Check sheet for the drawn part. Datum: minimum x, y, z corner. Units: mm. Round coordinates to 2 decimals unless told otherwise and drop trailing zeros. Order: outer loops, then holes, each group sorted by start corner. A loop starts at its lowest first (then second) coordinate and runs counter-clockwise, first axis right, second up. Notation, with made-up numbers: (-35.5, 80) -> (-15.5, 80) arc R9 ccw to (-15.5, 96) -> close; hole circle Ø8 at (56.5, -11.75). An arc over 180 degrees is marked (long way). Write item = value, one per line. Start each with the question number.
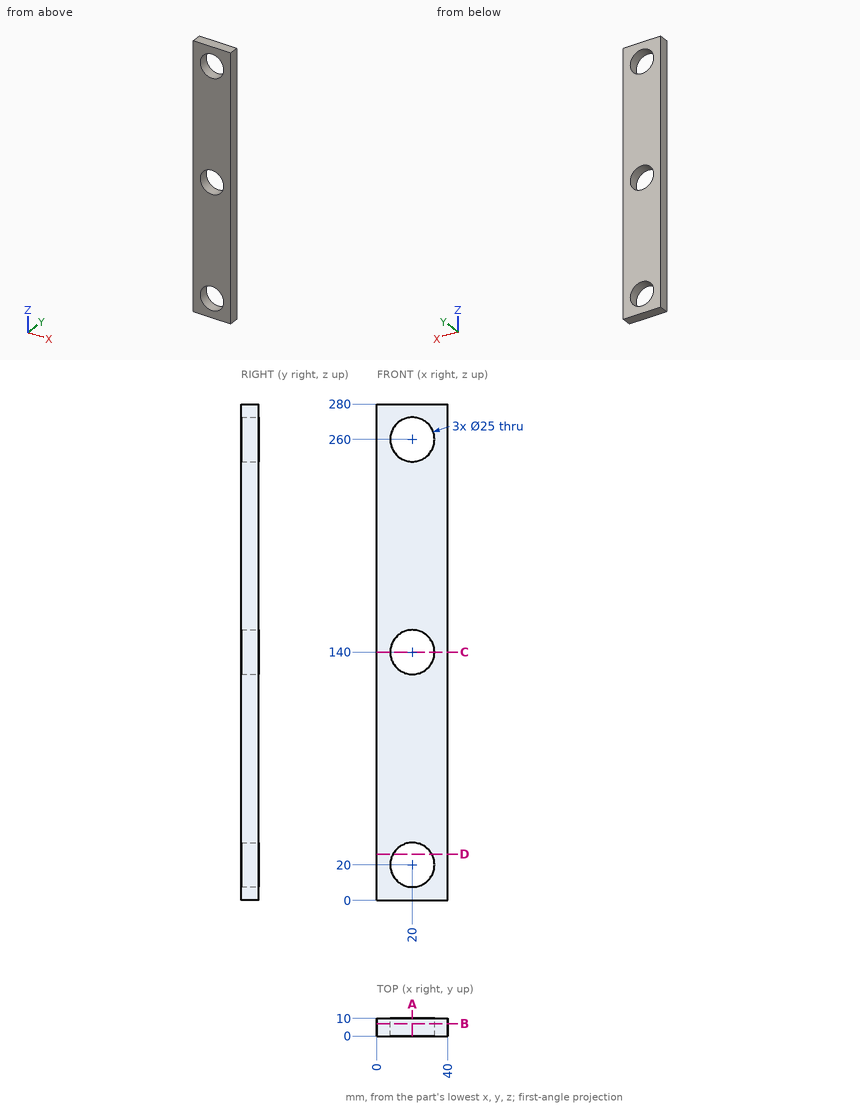
(1) Scan lines: line 1 along Z through (x, y) = (20, 3); line 2 along Z through (x, y) = (31, 2.5); line 3 along X through (y, z) = (7.75, 130). Record each from-to range of solid material in increasing order. Write a range as from..to.
(2) Cross-section at B-B (y = 7). Enter the section's corners in (x, z), and give its area (3 significant figures).
(3) Cross-section at C-C (z = 140). Enter the section's corners in (x, y), and give its area (3 significant figures).
(4) Cross-section at D-D (z = 26). Enter the section's corners in (x, y), and give its area (3 significant figures).
(5) Depth check by flat-ended pin: pin 1 (2 mm diameter, centred on x = 28.5, y = 8.5, fed in from -Z); pin 2 (20 mm diameter, centred on x = 20, z = 20, fed in from -Y). Enter the tip coordinate at first touch or a pass-through.
(6) Cross-section at A-A (x = 20). Enter the section's corners in (y, z), and give its area (3 significant figures).
Outcome:
q1.line_1 = 0..7.5, 32.5..127.5, 152.5..247.5, 272.5..280
q1.line_2 = 0..14.06, 25.94..134.06, 145.94..254.06, 265.94..280
q1.line_3 = 0..12.5, 27.5..40
q2.outline = (0, 0) -> (40, 0) -> (40, 280) -> (0, 280) -> close; hole circle Ø25 at (20, 20); hole circle Ø25 at (20, 140); hole circle Ø25 at (20, 260)
q2.area = 9,730 mm^2
q3.outline = (0, 0) -> (7.5, 0) -> (7.5, 10) -> (0, 10) -> close; (32.5, 0) -> (40, 0) -> (40, 10) -> (32.5, 10) -> close
q3.area = 150 mm^2
q4.outline = (0, 0) -> (9.03, 0) -> (9.03, 10) -> (0, 10) -> close; (30.97, 0) -> (40, 0) -> (40, 10) -> (30.97, 10) -> close
q4.area = 181 mm^2
q5.pin_1 = 0
q5.pin_2 = through
q6.outline = (0, 0) -> (10, 0) -> (10, 7.5) -> (0, 7.5) -> close; (0, 32.5) -> (10, 32.5) -> (10, 127.5) -> (0, 127.5) -> close; (0, 152.5) -> (10, 152.5) -> (10, 247.5) -> (0, 247.5) -> close; (0, 272.5) -> (10, 272.5) -> (10, 280) -> (0, 280) -> close
q6.area = 2,050 mm^2
